Autodesk Inventor part; units mm, degrees
ref_plane "YZ Plane" through (0, 0, 0) normal (1, 0, 0) x (0, 1, 0)
ref_plane "XZ Plane" through (0, 0, 0) normal (0, 1, 0) x (-1, 0, 0)
ref_plane "XY Plane" through (0, 0, 0) normal (0, 0, 1) x (1, 0, 0)
sketch "Sketch1" plane through (0, 0, 0) normal (0, 1, 0) x (-1, 0, 0)
  line L0 (0, 0) -> (7.62, 0)
  line L1 (7.62, 0) -> (7.62, -15.24)
  line L2 (7.62, -15.24) -> (0, -15.24)
  line L3 (0, -15.24) -> (0, 0)
  dimension "d0" = 7.62
  dimension "d1" = 15.24
extrude "Extrusion1" add sketch "Sketch1" along normal blind 1.905
sketch "Sketch4" plane through (0, 1.905, 0) normal (0, 1, 0) x (1, 0, 0)
  line L0 (0, 15.24) -> (-7.62, 15.24)
  circle A0 centre (-3.81, 11.43) radius 1.651
  point P0 (0, 0)
  point P1 (-3.81, 15.24)
  dimension "d9" = 3.302
  dimension "d10" = 3.81
extrude "Extrusion3" cut sketch "Sketch4" against normal through all
chamfer "Chamfer1" distance 1.27 angle 45 1 edges at (-5.461, 1.905, -11.43)
sketch "Sketch5" plane through (0, 1.905, 0) normal (0, 1, 0) x (1, 0, 0)
  line L0 (-7.62, 0) -> (0, 0)
  line L1 (0, 0) -> (0, 15.24)
  line L2 (0, 15.24) -> (-7.62, 15.24)
  line L3 (-7.62, 15.24) -> (-7.62, 0)
  circle A0 centre (-3.81, 11.43) radius 2.921
  line L4 (0, 0) -> (-7.62, 0)
  line L5 (-5.1435, 0) -> (-5.842, 0.9271)
  line L6 (-5.842, 0.9271) -> (-5.842, 1.6256)
  line L7 (-5.842, 1.6256) -> (-1.778, 1.6256)
  line L8 (-1.778, 1.6256) -> (-1.778, 0.9271)
  line L9 (-1.778, 0.9271) -> (-2.4765, 0)
  line L10 (-7.62, 0) -> (-7.62, 15.24)
  line L11 (-7.62, 3.81) -> (0, 3.81)
  point P0 (-3.81, 1.6256)
  point P1 (-3.81, 3.81)
  dimension "d19" = 2.667
  dimension "d20" = 4.064
  dimension "d21" = 0.9271
  dimension "d23" = 1.6256
  dimension "d24" = 3.81
extrude "Extrusion4" add sketch "Sketch5" along normal blind 3.175 contours L3 L11 L1 L0 L9 L8 L7 L6 L5
fillet "Fillet2" radius 1.27 6 edges at (-7.62, 2.54, 0) (0, 2.54, 0) (0, 3.4925, -3.81) (-7.62, 3.4925, -3.81) (-7.62, 0.9525, -15.24) (0, 0.9525, -15.24)
sketch "Sketch6" plane through (0, 1.905, 0) normal (0, 1, 0) x (1, 0, 0)
  line L0 (-2.4765, 0) -> (-1.778, 0.9271)
  line L1 (-1.778, 0.9271) -> (-1.778, 1.6256)
  line L2 (-1.778, 1.6256) -> (-5.842, 1.6256)
  line L3 (-5.842, 1.6256) -> (-5.842, 0.9271)
  line L4 (-5.842, 0.9271) -> (-5.1435, 0)
  line L5 (-5.1435, 0) -> (-2.4765, 0)
  point P0 (0, 0)
extrude "Extrusion5" cut sketch "Sketch6" against normal blind 1.016
properties part number "HallEffectSpoolSensorMount" material "ABS Plastic"
Input: part model. Units: mm. Frame: model coordinates. A direction names the side the tool comes from. Round coordinates to 2 decimals unless told otherwise and drop trailing zeros. Write each loop counter-clockwise with the first axis right and the second up, starting at its lowest first coordinate (ties: lowest second). Pieces come first, ordered by that corner, then holes.
1) Cut plane B-B (z = -11.43). Return the cut outline in (x, y) (3 decimals), then the cut area to 3 significant figures.
2) Reachability of faces 1 (the flat face through (-4, 3, -3.81)), 2 (the flat face through (-4, 3, -1.626)), 3 (the cylindrical face through (-7.238, 3.515, -3.448)) from +Z, -Z, +X, -X, +Y, -Y: full face, straight path, thin tool, end or side. Return the list, or none.
3) Cut plane C-C (y = 1.25). Return the cut outline in (x, z), then the cut area to 3 significant figures.
4) Cut plane D-D (y = 4.6). Return the cut outline in (x, z).
5) Contact query for flat-ended pins moving along their axis: P1, Ø0.8, axis at x = -4, z = -1, coming from the +Y side; P2, Ø2.5, axis at x = -2.5, z = -10.5, coming from the +Y side; P3, Ø1, axis at x = -3, y = 4, coming from the -Z side. Output: stop coordinate, or through.
6) Cut plane A-A (x = -3.81). Return the cut outline in (y, z) (3 decimals).
7) Draft query along X for faces 4 (the flat face through (0, 1, -6)), 5 (the flat face through (-4, 5.08, -2)), 6 (the flat face through (-5.49, 2.96, -0.46)). Return one class per face: pulls with the +X half, pulls with the -X half, needs draft (parallel to the pull), parting line crosses it, or undercut.
8) Ray query, L1, parallel to Z at x = -3.81, y = 0.2; L2, parallel to X at y = 0.25, z = -11.43; L3, parallel to Y at x = -3, z = -1.5. Return the intervals inside material, ascending.
Geometry says:
1. outline: (-7.62, 0) - (-5.461, 0) - (-5.461, 0.635) - (-6.731, 1.905) - (-7.62, 1.905) - close; (-2.159, 0) - (0, 0) - (0, 1.905) - (-0.889, 1.905) - (-2.159, 0.635) - close
1. area: 6.61 mm2
2. face 1: -Z, +X, -X, +Y
2. face 2: +Y
2. face 3: -Z, -X, +Y
3. outline: (-7.62, -13.97) arc R1.27 ccw to (-6.35, -15.24) - (-1.27, -15.24) arc R1.27 ccw to (0, -13.97) - (0, -1.27) arc R1.27 ccw to (-1.27, 0) - (-2.48, 0) - (-1.78, -0.93) - (-1.78, -1.63) - (-5.84, -1.63) - (-5.84, -0.93) - (-5.14, 0) - (-6.35, 0) arc R1.27 ccw to (-7.62, -1.27) - close; hole circle Ø4.53 at (-3.81, -11.43)
3. area: 92.7 mm2
4. outline: (-7.62, -2.54) arc R1.27 ccw to (-6.35, -3.81) - (-1.27, -3.81) arc R1.27 ccw to (0, -2.54) - (0, -1.27) arc R1.27 ccw to (-1.27, 0) - (-2.48, 0) - (-1.78, -0.93) - (-1.78, -1.63) - (-5.84, -1.63) - (-5.84, -0.93) - (-5.14, 0) - (-6.35, 0) arc R1.27 ccw to (-7.62, -1.27) - close
5. P1: stops at y = 0.89
5. P2: stops at y = 1.84
5. P3: stops at z = -3.81
6. outline: (0, -15.24) - (1.905, -15.24) - (1.905, -14.351) - (0.635, -13.081) - (0, -13.081) - close; (0, -9.779) - (0.635, -9.779) - (1.905, -8.509) - (1.905, -3.81) - (5.08, -3.81) - (5.08, -1.626) - (0.889, -1.626) - (0.889, 0) - (0, 0) - close
7. face 4: pulls with the +X half
7. face 5: needs draft
7. face 6: undercut
8. L1: z = -15.24 to -13.08, -9.78 to 0
8. L2: x = -7.62 to -5.46, -2.16 to 0
8. L3: y = 0 to 0.89
